Check sheet for the drawn part. Datum: minimum x, y, z corner. Units: mm. A direction names the side the tool comes from. Give positions to 0.01 mm unless a question says otherwise; leave off trailing zeros. Write each loop counter-clockwise with the first axis right and the second up, starting at its lowest first coordinate (ties: lowest second). Pieces come first, ordered by that corner, then holes.
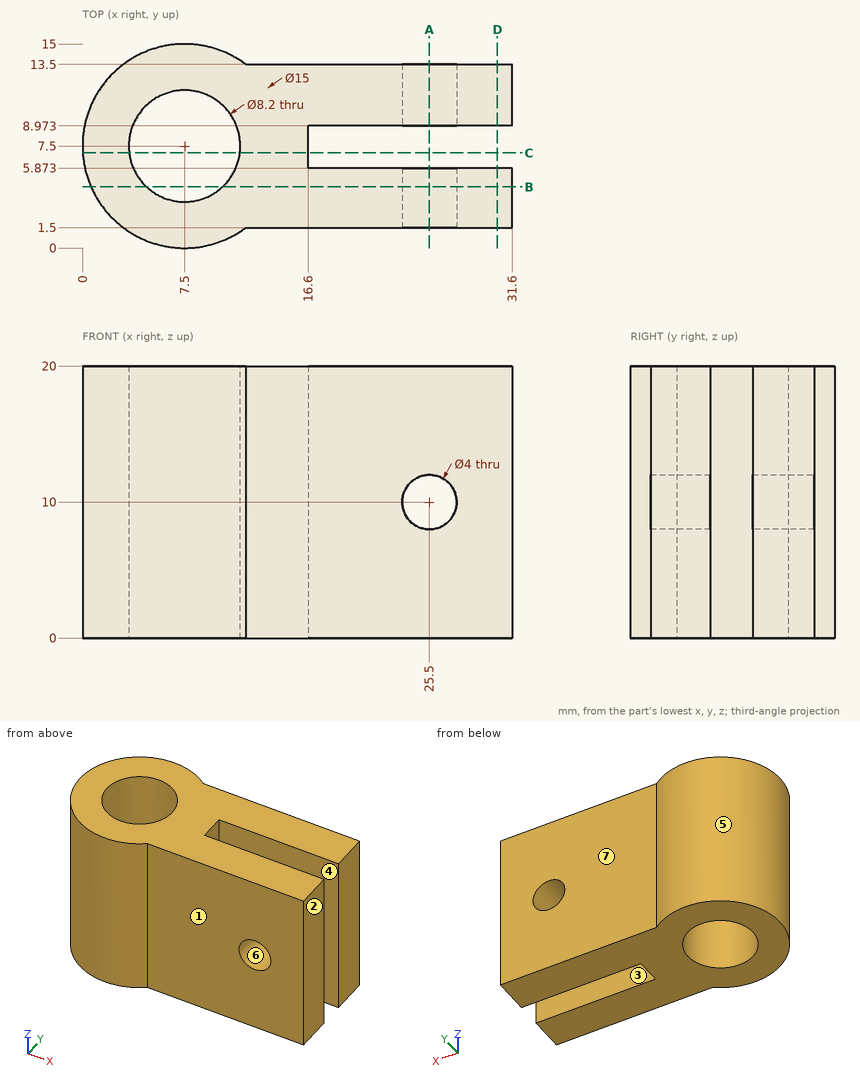
1) Sectioned sample at D-D on x = 30.5. Record the boundary of the cut face in (y, z), then the cut area to 3 significant figures.
2) Sectioned sample at A-A on x = 25.5. Record the boundary of the cut face in (y, z), then the cut area to 3 significant figures.
3) Access from +Z, -Z, +X, -X, +Y, -Y to the whole of each face (thin tool, end or side, straight path). Record for the marked faces 1, 2 and 3.
4) Sectioned sample at C-C on y = 7. Record the boundary of the cut face in (x, z).
5) Sectioned sample at B-B on y = 4.5. Record the boundary of the cut face in (x, z), then the cut area to 3 significant figures.
6) Draft check along Y on the marked faces 4, 5, 6 and 7. Enter one of: +Y half, -Y half, draft (parallel to the pull), parting line (faces both ways), or undercut.
7) Scan lines: L1, parallel to Z at x = 25.5, y = 11.1; L2, parallel to Y at x = 7.5, z = 6; L3, parallel to Y at x = 29, z = 1. Record each from-to range of solid material in increasing order.
8) Gauge pin test, flat ends, axial feed: pin 1 (6 mm diameter, centred on x = 24.5, z = 13.5, fed in from +Y); pin 2 (7.5 mm diameter, centred on x = 24, z = 12, fed in from -Y); pin 3 (1.5 mm diameter, centred on x = 6.5, z = 14.5, fed in from -Y); pin 4 (3 mm diameter, centred on x = 25.5, z = 10, fed in from +Y) (3 decimals). Record the tip position at first contact, or that the pin passes through.
Answers below:
1. outline: (1.5, 0) - (5.87, 0) - (5.87, 20) - (1.5, 20) - close; (8.97, 0) - (13.5, 0) - (13.5, 20) - (8.97, 20) - close
1. area: 178 mm2
2. outline: (1.5, 0) - (5.87, 0) - (5.87, 8) - (1.5, 8) - close; (1.5, 12) - (5.87, 12) - (5.87, 20) - (1.5, 20) - close; (8.97, 0) - (13.5, 0) - (13.5, 8) - (8.97, 8) - close; (8.97, 12) - (13.5, 12) - (13.5, 20) - (8.97, 20) - close
2. area: 142 mm2
3. face 1: +Z, -Z, +X, -Y
3. face 2: +Z, -Z, +X, +Y, -Y
3. face 3: +Z, -Z, +X
4. outline: (0.02, 0) - (3.43, 0) - (3.43, 20) - (0.02, 20) - close; (11.57, 0) - (16.6, 0) - (16.6, 20) - (11.57, 20) - close
5. outline: (0.63, 0) - (4.71, 0) - (4.71, 20) - (0.63, 20) - close; (10.29, 0) - (31.6, 0) - (31.6, 20) - (10.29, 20) - close; hole circle Ø4 at (25.5, 10)
5. area: 495 mm2
6. face 4: undercut
6. face 5: parting line
6. face 6: draft
6. face 7: +Y half
7. L1: z = 0 to 8, 12 to 20
7. L2: y = 0 to 3.4, 11.6 to 15
7. L3: y = 1.5 to 5.87, 8.97 to 13.5
8. pin 1: stops at y = 13.5
8. pin 2: stops at y = 1.5
8. pin 3: stops at y = 0
8. pin 4: passes through
